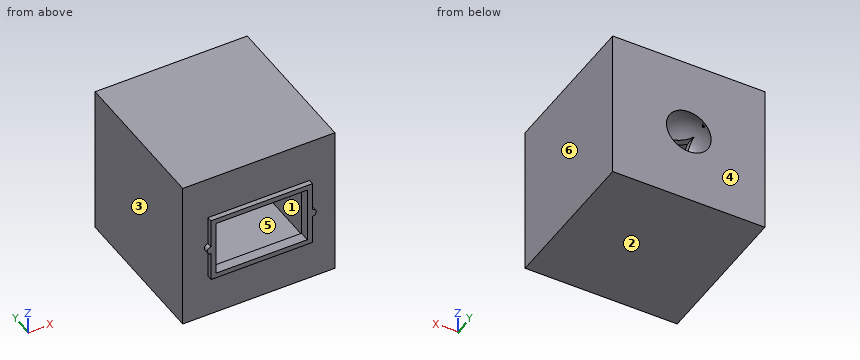
```python
from build123d import *

# Parameters (mm, degrees)
SKETCH1_W                  = 76.2
SKETCH1_H                  = 76.2
MAIN_BODY_DEPTH            = 76.2
SKETCH6_W                  = 50.8
SKETCH6_H                  = 33.02
CAMERA_BASE_DEPTH          = 2.54
SHELL_T                    = -2.54
SKETCH13_R                 = 1.905
SCREW_MOUNTS_DEPTH         = 2.54
F_4_40_TAPPED_HOLE1_REACH  = 95.326
F_4_40_TAPPED_HOLE1_BORE_R = 1.1303
CHECK_OUT_THE_BOTTOM_REACH = 95.326
SKETCH16_W                 = 19.05
SKETCH16_H                 = 19.05


with BuildPart() as part:
    # Sketch1 → main body (new body)
    with BuildSketch(Plane(origin=(0, 0, 0), x_dir=(1, 0, 0), z_dir=(0, 1, 0))):
        Rectangle(SKETCH1_W, SKETCH1_H)
    extrude(amount=MAIN_BODY_DEPTH)

    # Sketch5 → trackball hole (revolve, cut)
    with BuildSketch(Plane.XY):
        with BuildLine():
            Line((0, 81.788), (0, 53.848))
            ThreePointArc((0, 53.848), (13.97, 67.818), (0, 81.788))
        make_face()
    revolve(axis=Axis((0, -906.782, 0), (0, 1, 0)), mode=Mode.SUBTRACT)

    # Sketch6 → camera base (add)
    with BuildSketch(Plane.XZ):
        Rectangle(SKETCH6_W, SKETCH6_H)
    extrude(amount=CAMERA_BASE_DEPTH)

    # shell
    shell_openings = [part.faces().sort_by_distance(p)[0] for p in [
        (0, -2.54, 0),
    ]]
    offset(amount=SHELL_T, openings=shell_openings, kind=Kind.INTERSECTION)

    # Sketch13 → screw mounts (add)
    with BuildSketch(Plane.XZ):
        with Locations((-25.4, 0)):
            Circle(SKETCH13_R)
        with Locations((25.4, 0)):
            Circle(SKETCH13_R)
    extrude(amount=SCREW_MOUNTS_DEPTH)

    # #4-40 Tapped Hole1 bore → #4-40 Tapped Hole1 (cut, up to next)
    with BuildSketch(Plane(origin=(0, 0, 0), x_dir=(-1, 0, 0), z_dir=(0, -1, 0)), mode=Mode.PRIVATE) as f_4_40_tapped_hole1_sk1:
        with Locations((25.4, 0)):
            Circle(F_4_40_TAPPED_HOLE1_BORE_R)
    f_4_40_tapped_hole1_tool1 = extrude(f_4_40_tapped_hole1_sk1.sketch, amount=-F_4_40_TAPPED_HOLE1_REACH, mode=Mode.PRIVATE) & part.part
    # #4-40 Tapped Hole1 bore → #4-40 Tapped Hole1 (cut, up to next)
    with BuildSketch(Plane(origin=(0, 0, 0), x_dir=(-1, 0, 0), z_dir=(0, -1, 0)), mode=Mode.PRIVATE) as f_4_40_tapped_hole1_sk2:
        with Locations((-25.4, 0)):
            Circle(F_4_40_TAPPED_HOLE1_BORE_R)
    f_4_40_tapped_hole1_tool2 = extrude(f_4_40_tapped_hole1_sk2.sketch, amount=-F_4_40_TAPPED_HOLE1_REACH, mode=Mode.PRIVATE) & part.part
    add(f_4_40_tapped_hole1_tool1.solids().sort_by_distance((-25.4, 0, 0))[0], mode=Mode.SUBTRACT)
    add(f_4_40_tapped_hole1_tool2.solids().sort_by_distance((25.4, 0, 0))[0], mode=Mode.SUBTRACT)

    # check out the bottom: up to this face of the body (flat: up to its plane)
    check_out_the_bottom_end = Plane(part.part.faces().sort_by_distance((0, 73.66, -34.554211314))[0])
    # Sketch16 → check out the bottom (cut, up to the picked face)
    with BuildSketch(Plane(origin=(0, 0, 0), x_dir=(1, 0, 0), z_dir=(0, 1, 0)), mode=Mode.PRIVATE) as check_out_the_bottom_sk1:
        Rectangle(SKETCH16_W, SKETCH16_H)
    check_out_the_bottom_tool1 = split(extrude(check_out_the_bottom_sk1.sketch, amount=CHECK_OUT_THE_BOTTOM_REACH, mode=Mode.PRIVATE), bisect_by=check_out_the_bottom_end, keep=Keep.BOTH, mode=Mode.PRIVATE)
    add(check_out_the_bottom_tool1.solids().sort_by(Axis((0, 0, 0), (0, 1, 0)))[0], mode=Mode.SUBTRACT)


solid = part.part
```
Work out the finished part from the listing and answer in its coordinate system (mm). Face numbers are marked on the shaded views. A direction names the side the tool comes from. Coordinates: 2 decimals unless noted, no trailing zeros. Order: outer loops, then holes, each group sorted by start corner. A loop starts at its lowest first (then second) coordinate and runs counter-clockwise, first axis right, second up. Notation, with made-up numbers: (66.25, 39.25) - (80.25, 39.25) arc R26 cw to (80.25, 66.25) - close; hole circle Ø9 at (1, -29). An arc over 180 degrees is marked (long way). Answer as a JSON object with one key per item and string values.
1. The mould has two halves that part along X. Classify the marked faces 3, 4, 5 and 6: +X half, -X half, draft (parallel to the pull), parting line (faces both ways), or undercut.
Output values:
{"face 3": "-X half", "face 4": "draft", "face 5": "undercut", "face 6": "+X half"}
2. Find section C-C on y = 61. Determine the outline of the cut face in (x, z) (1 decimal), plus the area to 3 significant figures.
Output values:
{"outline": "(-38.1, -38.1) - (38.1, -38.1) - (38.1, 38.1) - (-38.1, 38.1) - close; circle Ø30.1 at (0, 0); hole (-35.6, -35.6) - (35.6, -35.6) - (35.6, 35.6) - (-35.6, 35.6) - close; hole (-9.5, -9.5) - (-7.6, -9.5) arc R12.2 ccw to (7.6, -9.5) - (9.5, -9.5) - (9.5, -7.6) arc R12.2 ccw to (9.5, 7.6) - (9.5, 9.5) - (7.6, 9.5) arc R12.2 ccw to (-7.6, 9.5) - (-9.5, 9.5) - (-9.5, 7.6) arc R12.2 ccw to (-9.5, -7.6) - close", "area": "985 mm²"}
3. A tool of negligible diameter and unlimited length cuts with its end or side. For the marked faces 1 and 2, from which of +Z, -Z, +X, -X, +Y, -Y can it reach the whole face along a straight path? Write none if from no direction.
Output values:
{"face 1": "none", "face 2": "-Z, +X, -X, +Y, -Y"}
4. Find section A-A on x = 29. Determine the outline of the cut face in (y, z).
Output values:
{"outline": "(0, -38.1) - (76.2, -38.1) - (76.2, 38.1) - (0, 38.1) - close; hole (2.54, -35.56) - (73.66, -35.56) - (73.66, 35.56) - (2.54, 35.56) - close"}
5. Find section B-B on z = 23.5. Determine the outline of the cut face in (x, y).
Output values:
{"outline": "(-38.1, 0) - (38.1, 0) - (38.1, 76.2) - (-38.1, 76.2) - close; hole (-35.56, 2.54) - (35.56, 2.54) - (35.56, 73.66) - (-35.56, 73.66) - close"}
6. Consider line 1 (X direction, y = 1.2, z = 0); line 2 (Z direction, x = 14.5, y = 18); line 3 (Y direction, x = -23.5, z = 22). Determine where each line is inside the solid, lowest interval first.
Output values:
{"line 1": "x = -38.1 to -26.53, -24.27 to -22.86, 22.86 to 24.27, 26.53 to 38.1", "line 2": "z = -38.1 to -35.56, 35.56 to 38.1", "line 3": "y = 0 to 2.54, 73.66 to 76.2"}
7. Each of these flat-tipped pins is pushed along its axis until it touches: P1, Ø0.8, axis at y = -1, z = 7, coming from the +X side; P2, Ø0.9, axis at x = -9, z = 9, coming from the -Y side; P3, Ø0.8, axis at x = 6.5, y = -0.5, coming from the -Z side; P4, Ø3, axis at x = -7, z = 2.5, coming from the +Y side. Where does it stop, or does it pass through?
Output values:
{"P1": "stops at x = 25.4", "P2": "stops at y = 73.66", "P3": "stops at z = -16.51", "P4": "passes through"}
